Geometry check sheet. Reference: the model listing, model coordinates, mm. Face numbers are marked on the shaded views. Round coordinates to 2 decimals unless told otherwise and drop trailing zeros. Order: outer loops, then holes, each group sorted by start corner. A loop starts at its lowest first (then second) coordinate and runs counter-clockwise, first axis right, second up. Notation, with made-up numbers: (33, 12) -> (48, 12) arc R30 cw to (48, 39) -> close; hole circle Ø8 at (67.25, 88). An arc over 180 degrees is marked (long way). Use a Markdown table: item, result. Add a question column.
Item 1: Sectioned sample at C-C, the plane z = -4.5. Record the cut outline in (x, y), and give its area (3 significant figures).
Item 2: Sectioned sample at B-B, the plane z = 0. Record the cut outline in (x, y), and give its area (3 significant figures).
Item 3: Material ranges on probe 1 along X at (y, z) = (2.5, 0); probe 2 along Y at (x, z) = (1, 6.25); probe 3 along X at (y, z) = (4.75, -1.5), recorded low to high. Write a range as [from, to].
Item 4: Mould release check, pull along X, two halves, no side actions. Record for the marked faces 1, 2 and 3: pulls with the +X half, pulls with the -X half, needs draft (parallel to the pull), parting line crosses it, or undercut.
Item 5: Sectioned sample at A-A, the plane x = 0. Record the cut outline in (y, z), and give its area (3 significant figures).
Item 6: Sectioned sample at D-D, the plane y = 2.5. Record the cut outline in (x, z).
Item 7: Gauge pin test, flat ends, axial feed: pin 1 Ø1.5 at (x, z) = (5, 5) entering from +Y; pin 2 Ø5 at (x, z) = (2.5, -1) entering from -Y; pin 3 Ø3 at (x, y) = (0.5, 5.5) entering from -Z. Record the tip position at first contact, or that the pin passes through.
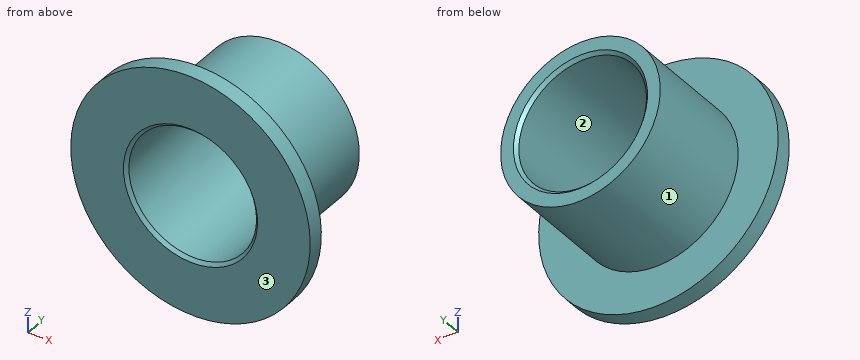
from build123d import *

# Parameters (mm, degrees)
SKIZZE1_R                       = 7.5
AUFSATZ_LINEAR_AUSTRAGEN1_DEPTH = 1
SKIZZE2_R                       = 5
AUFSATZ_LINEAR_AUSTRAGEN2_DEPTH = 7
SKIZZE4_R                       = 4
SCHNITT_LINEAR_AUSTRAGEN1_DEPTH = 14.285330256
FASE1_SIZE                      = 0.2


with BuildPart() as part:
    # Skizze1 → Aufsatz-Linear austragen1 (new body)
    with BuildSketch(Plane(origin=(0, 0, 0), x_dir=(1, 0, 0), z_dir=(0, 1, 0))):
        with Locations(Location((0, 0, 0), (0, 0, 270))):
            Circle(SKIZZE1_R)
    extrude(amount=AUFSATZ_LINEAR_AUSTRAGEN1_DEPTH)

    # Skizze2 → Aufsatz-Linear austragen2 (add)
    with BuildSketch(Plane(origin=(0, 1, 0), x_dir=(1, 0, 0), z_dir=(0, 1, 0))):
        with Locations(Location((0, 0, 0), (0, 0, 270))):
            Circle(SKIZZE2_R)
    extrude(amount=AUFSATZ_LINEAR_AUSTRAGEN2_DEPTH)

    # Skizze4 → Schnitt-Linear austragen1 (cut, through all)
    with BuildSketch(Plane(origin=(0, 8, 0), x_dir=(1, 0, 0), z_dir=(0, 1, 0))):
        with Locations(Location((0, 0, 0), (0, 0, 270))):
            Circle(SKIZZE4_R)
    extrude(amount=-SCHNITT_LINEAR_AUSTRAGEN1_DEPTH, mode=Mode.SUBTRACT)

    # Fase1
    fase1_edges = [part.edges().sort_by_distance(p)[0] for p in [
        (0, 0, -4),
        (0, 8, -4),
    ]]
    chamfer(fase1_edges, length=FASE1_SIZE)


solid = part.part
Found:
| question | item | result |
|---|---|---|
| 1 | outline | (-6, 0) -> (6, 0) -> (6, 1) -> (2.18, 1) -> (2.18, 8) -> (-2.18, 8) -> (-2.18, 1) -> (-6, 1) -> close |
| 1 | area | 42.5 mm2 |
| 2 | outline | (-7.5, 0) -> (-4.2, 0) -> (-4, 0.2) -> (-4, 7.8) -> (-4.2, 8) -> (-5, 8) -> (-5, 1) -> (-7.5, 1) -> close; (4, 0.2) -> (4.2, 0) -> (7.5, 0) -> (7.5, 1) -> (5, 1) -> (5, 8) -> (4.2, 8) -> (4, 7.8) -> close |
| 2 | area | 20.9 mm2 |
| 3 | probe 1 | x = [-5, -4], [4, 5] |
| 3 | probe 2 | y = [0, 1] |
| 3 | probe 3 | x = [-4.77, -3.71], [3.71, 4.77] |
| 4 | face 1 | parting line crosses it |
| 4 | face 2 | undercut |
| 4 | face 3 | needs draft |
| 5 | outline | (0, -7.5) -> (1, -7.5) -> (1, -5) -> (8, -5) -> (8, -4.2) -> (7.8, -4) -> (0.2, -4) -> (0, -4.2) -> close; (0, 4.2) -> (0.2, 4) -> (7.8, 4) -> (8, 4.2) -> (8, 5) -> (1, 5) -> (1, 7.5) -> (0, 7.5) -> close |
| 5 | area | 20.9 mm2 |
| 6 | outline | circle Ø10 at (0, 0); hole circle Ø8 at (0, 0) |
| 7 | pin 1 | stops at y = 1 |
| 7 | pin 2 | stops at y = 0 |
| 7 | pin 3 | stops at z = -5 |
